```python
from build123d import *

# Parameters (mm, degrees)
SKETCH1_W            = 390
SKETCH1_H            = 756.8
BOSS_EXTRUDE1_DEPTH  = 20
SKETCH2_R            = 6.05
BOSS_EXTRUDE2_DEPTH  = 10
SKETCH3_R            = 6.631048811
BOSS_EXTRUDE3_DEPTH  = 10
CHAMFER1_SIZE        = 10
BOSS_EXTRUDE5_DEPTH  = 50
SKETCH5_W            = 30
SKETCH5_H            = 160
CUT_EXTRUDE1_DEPTH   = 50
CHAMFER2_SIZE        = 10
CUT_EXTRUDE2_DEPTH   = 121
SKETCH10_W           = 25
SKETCH10_H           = 25
BOSS_EXTRUDE7_DEPTH  = 8
SKETCH15_W           = 19.321199796
SKETCH15_H           = 9.52453511
BOSS_EXTRUDE8_DEPTH  = 40
SKETCH16_W           = 18.085272723
SKETCH16_H           = 9.99449282
BOSS_EXTRUDE9_DEPTH  = 40
SKETCH18_W           = 18.812893718
SKETCH18_H           = 136.043392328
BOSS_EXTRUDE10_DEPTH = 10
FILLET1_R            = 2
FILLET2_R            = 2
FILLET3_R            = 2
CUT_EXTRUDE3_START   = -10
SKETCH23_R           = 6.05
CUT_EXTRUDE3_DEPTH   = 10
SKETCH24_R           = 7.299940413
BOSS_EXTRUDE11_DEPTH = 1
BOSS_EXTRUDE12_START = 10
SKETCH27_R           = 6.63104881
BOSS_EXTRUDE12_DEPTH = 10


with BuildPart() as part:
    # Sketch1 → Boss-Extrude1 (new body)
    with BuildSketch(Plane.XY):
        with Locations((154.409313495, -346.327898551)):
            Rectangle(SKETCH1_W, SKETCH1_H)
    extrude(amount=BOSS_EXTRUDE1_DEPTH)

    # Sketch2 → Boss-Extrude2 (add)
    with BuildSketch(Plane(origin=(0, 32.072101449, 0), x_dir=(1, 0, 0), z_dir=(0, 1, 0))):
        with Locations(Location((-28.78378628, -10.435138004, 0), (0, 0, 90))):
            Circle(SKETCH2_R)
    extrude(amount=BOSS_EXTRUDE2_DEPTH)

    # Sketch3 → Boss-Extrude3 (add)
    with BuildSketch(Plane.XZ.offset(724.727898551)):
        with Locations(Location((-28.78378628, 10.435138004, 0), (0, 0, 90))):
            Circle(SKETCH3_R)
    extrude(amount=BOSS_EXTRUDE3_DEPTH)

    # Chamfer1
    # the kernel refuses this chamfer: 10 mm, written as the material it takes off along each edge
    with BuildSketch(Plane(origin=(-40.590686505, -750.44472843, 20), x_dir=(-0.027495876610586317, 0, -0.9996219169112968), z_dir=(0, 1, 0)), Plane(origin=(349.409313495, 57.788931329, 0), x_dir=(-0.9996219169112968, 0, -0.027495876610586334), z_dir=(0, -1, 0))) as chamfer1_piece_1:
        Polygon((CHAMFER1_SIZE * 0.999621916911, -CHAMFER1_SIZE * 0.0274958766106), (-CHAMFER1_SIZE * 0.0274958766106, -CHAMFER1_SIZE * 0.999621916911), (0, 0), align=None)
    extrude(amount=808.233659759, mode=Mode.SUBTRACT)
    with BuildSketch(Plane(origin=(375.126143374, -724.727898551, 20), x_dir=(0, 0.9996219169112968, 0.02749587661058643), z_dir=(-1, 0, 0))) as chamfer1_piece_2_section:
        Polygon((CHAMFER1_SIZE * 0.999621916911, CHAMFER1_SIZE * 0.0274958766106), (-CHAMFER1_SIZE * 0.0274958766106, CHAMFER1_SIZE * 0.999621916911), (0, 0), align=None)
    chamfer1_piece_2 = extrude(amount=441.433659759, mode=Mode.PRIVATE)
    chamfer1_piece_2 = chamfer1_piece_2 - Plane(origin=(-28.78378628, -721.415314621, 10.435138004), x_dir=(0, 0, 1), z_dir=(0, 1, 0)) * Cylinder(6.631048811, 923, mode=Mode.PRIVATE)
    add(chamfer1_piece_2, mode=Mode.SUBTRACT)
    with BuildSketch(Plane(origin=(349.409313495, 57.788931329, 20), x_dir=(-0.9996219169112968, 0, 0.027495876610586282), z_dir=(0, -1, 0)), Plane(origin=(-40.590686505, -750.44472843, 0), x_dir=(-0.027495876610586317, 0, 0.9996219169112968), z_dir=(0, 1, 0))) as chamfer1_piece_3:
        Polygon((CHAMFER1_SIZE * 0.999621916911, CHAMFER1_SIZE * 0.0274958766106), (-CHAMFER1_SIZE * 0.0274958766106, CHAMFER1_SIZE * 0.999621916911), (0, 0), align=None)
    extrude(amount=808.233659759, mode=Mode.SUBTRACT)
    with BuildSketch(Plane(origin=(-66.307516385, 32.072101449, 20), x_dir=(0, 0.027495876610586317, -0.9996219169112968), z_dir=(1, 0, 0))) as chamfer1_piece_4_section:
        Polygon((CHAMFER1_SIZE * 0.999621916911, -CHAMFER1_SIZE * 0.0274958766106), (-CHAMFER1_SIZE * 0.0274958766106, -CHAMFER1_SIZE * 0.999621916911), (0, 0), align=None)
    chamfer1_piece_4 = extrude(amount=441.433659759, mode=Mode.PRIVATE)
    chamfer1_piece_4 = chamfer1_piece_4 - Plane(origin=(-28.78378628, 28.76135635, 10.435138004), x_dir=(0, 0, -1), z_dir=(0, -1, 0)) * Cylinder(6.05, 923, mode=Mode.PRIVATE)
    add(chamfer1_piece_4, mode=Mode.SUBTRACT)
    with BuildSketch(Plane(origin=(375.126143374, -724.727898551, 0), x_dir=(0, 0.9996219169112968, -0.027495876610586487), z_dir=(-1, 0, 0))) as chamfer1_piece_5_section:
        Polygon((CHAMFER1_SIZE * 0.999621916911, -CHAMFER1_SIZE * 0.0274958766106), (-CHAMFER1_SIZE * 0.0274958766106, -CHAMFER1_SIZE * 0.999621916911), (0, 0), align=None)
    chamfer1_piece_5 = extrude(amount=441.433659759, mode=Mode.PRIVATE)
    chamfer1_piece_5 = chamfer1_piece_5 - Plane(origin=(-28.78378628, -721.416873801, 10.435138004), x_dir=(0, 0, 1), z_dir=(0, 1, 0)) * Cylinder(6.631048811, 923, mode=Mode.PRIVATE)
    add(chamfer1_piece_5, mode=Mode.SUBTRACT)
    with BuildSketch(Plane(origin=(-66.307516385, 32.072101449, 0), x_dir=(0, 0.027495876610586317, 0.9996219169112968), z_dir=(1, 0, 0))) as chamfer1_piece_6_section:
        Polygon((CHAMFER1_SIZE * 0.999621916911, CHAMFER1_SIZE * 0.0274958766106), (-CHAMFER1_SIZE * 0.0274958766106, CHAMFER1_SIZE * 0.999621916911), (0, 0), align=None)
    chamfer1_piece_6 = extrude(amount=441.433659759, mode=Mode.PRIVATE)
    chamfer1_piece_6 = chamfer1_piece_6 - Plane(origin=(-28.78378628, 28.763199232, 10.435138004), x_dir=(0, 0, -1), z_dir=(0, -1, 0)) * Cylinder(6.05, 923, mode=Mode.PRIVATE)
    add(chamfer1_piece_6, mode=Mode.SUBTRACT)

    # Sketch4 → Boss-Extrude5 (add)
    with BuildSketch(Plane.XY.offset(20)):
        Polygon((309.409313495, -346.327898551), (309.409313495, -246.327898551), (339.409313495, -246.327898551), (339.409313495, -446.327898551), (309.409313495, -446.327898551), align=None)
    extrude(amount=BOSS_EXTRUDE5_DEPTH)

    # Sketch5 → Cut-Extrude1 (cut)
    with BuildSketch(Plane(origin=(339.409313495, 0, 0), x_dir=(0, 0, -1), z_dir=(1, 0, 0))):
        with Locations((-35, -346.327898551)):
            Rectangle(SKETCH5_W, SKETCH5_H)
    extrude(amount=-CUT_EXTRUDE1_DEPTH, mode=Mode.SUBTRACT)

    # Chamfer2
    chamfer2_edges = [part.edges().sort_by_distance(p)[0] for p in [
        (309.409313495, -346.327898551, 70),
        (309.409313495, -246.327898551, 45),
        (324.409313495, -446.327898551, 70),
        (309.409313495, -446.327898551, 45),
        (339.409313495, -446.327898551, 45),
        (324.409313495, -246.327898551, 70),
        (339.409313495, -246.327898551, 45),
        (339.409313495, -346.327898551, 70),
    ]]
    chamfer(chamfer2_edges, length=CHAMFER2_SIZE)

    # Sketch7 → Cut-Extrude2 (cut)
    with BuildSketch(Plane.XY.offset(20)):
        Polygon((309.409313495, -256.327898551), (319.409313495, -246.327898551), (329.409313495, -246.327898551), (339.409313495, -256.327898551), (339.409313495, -436.327898551), (329.409313495, -446.327898551), (319.409313495, -446.327898551), (309.409313495, -436.327898551), align=None)
    extrude(amount=CUT_EXTRUDE2_DEPTH, mode=Mode.SUBTRACT)

    # Sketch10 → Boss-Extrude7 (add)
    with BuildSketch(Plane.XY.offset(20)):
        with Locations((311.909313495, -240.427898551)):
            Rectangle(SKETCH10_W, SKETCH10_H)
        with Locations((311.909313495, -365.427898551)):
            Rectangle(SKETCH10_W, SKETCH10_H)
    extrude(amount=BOSS_EXTRUDE7_DEPTH)

    # Sketch15 → Boss-Extrude8 (add)
    with BuildSketch(Plane.XY.offset(28)):
        with Locations((311.88508976, -239.60936129)):
            Rectangle(SKETCH15_W, SKETCH15_H)
    extrude(amount=BOSS_EXTRUDE8_DEPTH)

    # Sketch16 → Boss-Extrude9 (add)
    with BuildSketch(Plane.XY.offset(28)):
        with Locations((311.994747219, -365.893239653)):
            Rectangle(SKETCH16_W, SKETCH16_H)
    extrude(amount=BOSS_EXTRUDE9_DEPTH)

    # Sketch18 → Boss-Extrude10 (add)
    with BuildSketch(Plane.XY.offset(68)):
        with Locations((311.630936721, -302.868789899)):
            Rectangle(SKETCH18_W, SKETCH18_H)
    extrude(amount=BOSS_EXTRUDE10_DEPTH)

    # Fillet1
    fillet1_edges = [part.edges().sort_by_distance(p)[0] for p in [
        (302.224489862, -307.631057454, 68),
        (321.03738358, -302.633811044, 68),
        (321.03738358, -302.868789899, 78),
        (302.224489862, -302.868789899, 78),
    ]]
    fillet(fillet1_edges, radius=FILLET1_R)

    # Fillet2
    fillet2_edges = [part.edges().sort_by_distance(p)[0] for p in [
        (299.409313495, -240.427898551, 28),
        (311.909313495, -252.927898551, 28),
        (324.409313495, -240.427898551, 28),
        (311.909313495, -227.927898551, 28),
    ]]
    fillet(fillet2_edges, radius=FILLET2_R)

    # Fillet3
    fillet3_edges = [part.edges().sort_by_distance(p)[0] for p in [
        (299.409313495, -365.427898551, 28),
        (311.909313495, -377.927898551, 28),
        (324.409313495, -365.427898551, 28),
        (311.909313495, -352.927898551, 28),
    ]]
    fillet(fillet3_edges, radius=FILLET3_R)

    # Sketch23 → Cut-Extrude3 (cut)
    with BuildSketch(Plane(origin=(0, 42.072101449, 0), x_dir=(1, 0, 0), z_dir=(0, 1, 0)).offset(CUT_EXTRUDE3_START)):
        with Locations((-28.78378628, -10.435138004)):
            Circle(SKETCH23_R)
    extrude(amount=CUT_EXTRUDE3_DEPTH, mode=Mode.SUBTRACT)

    # Sketch24 → Boss-Extrude11 (add)
    with BuildSketch(Plane(origin=(0, 32.072101449, 0), x_dir=(1, 0, 0), z_dir=(0, 1, 0))):
        with Locations((-28.78378628, -10.435138004)):
            Circle(SKETCH24_R)
    extrude(amount=-BOSS_EXTRUDE11_DEPTH)

    # Sketch27 → Boss-Extrude12 (add)
    with BuildSketch(Plane(origin=(0, 32.072101449, 0), x_dir=(1, 0, 0), z_dir=(0, 1, 0)).offset(BOSS_EXTRUDE12_START)):
        with Locations(Location((-28.78378628, -10.435138004, 0), (0, 0, 3.762526837))):
            Circle(SKETCH27_R)
    extrude(amount=-BOSS_EXTRUDE12_DEPTH)


solid = part.part
```
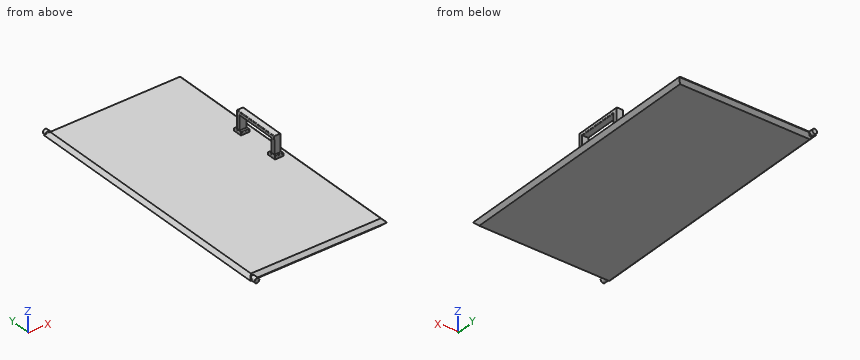
For this review, take the finished solid that the model builds, in its own axes (mm). Round coordinates to 2 decimals unless told otherwise and drop trailing zeros. Write each loop counter-clockwise with the first axis right and the second up, starting at its lowest first coordinate (ties: lowest second). Pieces come first, ordered by that corner, then holes. Notation, with made-up numbers: (-9.75, 64) - (-4.75, 64) arc R10 ccw to (-4.75, 76) - close; hole circle Ø5 at (-18.5, -1). An arc over 180 degrees is marked (long way). Answer as a JSON object with one key per item and string values.
1. We need section C-C on y = -453.5. Give the boundary of the cut face in (x, z).
Response values:
{"outline": "(-40.59, 10) - (-30.59, 0) - (339.41, 0) - (349.41, 10) - (339.41, 20) - (-30.59, 20) - close"}
2. To check wall thickness, follow line 1 along Z through (x, y) = (312.5, -285); line 2 along Z through (x, y) = (163.5, -571); line 3 along X through (y, z) = (-364, 26). State the ranges of each line that lie inside material, in increasing order.
Response values:
{"line 1": "z = 0 to 20, 68 to 78", "line 2": "z = 0 to 20", "line 3": "x = 299.41 to 324.41"}
3. We need section B-B on x = 47.5. Give the boundary of the cut face in (y, z), then the cut area to 3 significant figures.
Response values:
{"outline": "(-724.73, 10) - (-714.73, 0) - (22.07, 0) - (32.07, 10) - (22.07, 20) - (-714.73, 20) - close", "area": "14,900 mm2"}
4. For pin 1 Ø4 at (x, y) = (249.5, -527.5) entering from +Z; pin 2 Ø10.5 at (y, z) = (-239.5, 56.5) entering from +X; pin 3 Ø1.8 at (x, z) = (313, 22.5) entering from -Y; pin 4 Ø24 at (y, z) = (-316, 49) entering from -X, all flat-tipped, find the tip position at first contact; note any pin that passes through.
Response values:
{"pin 1": "stops at z = 20", "pin 2": "stops at x = 321.55", "pin 3": "stops at y = -377.93", "pin 4": "passes through"}
5. We need section A-A on z = 46. Give the boundary of the cut face in (x, y).
Response values:
{"outline": "(302.22, -244.37) - (321.55, -244.37) - (321.55, -234.85) - (302.22, -234.85) - close; (302.95, -370.89) - (321.04, -370.89) - (321.04, -360.9) - (302.95, -360.9) - close"}
